Verification items for this drawing (mm, ordinates from the low corner). A direction names the side the tool comes from. Round coordinates to 2 decimals unless told otherwise and drop trailing zeros. Loops run counter-clockwise (first coordinate to the right, second up) from the corner with the lowest first, then second, coordinate; pieces in that order, holes last. Notation, with made-up numbers: M 83.5,6.5 L 87.5,6.5 A20 ccw 87.5,11.5 Z; hole C 32,13 d4. An arc over 180 degrees is marked long. One line per item, written item: value.
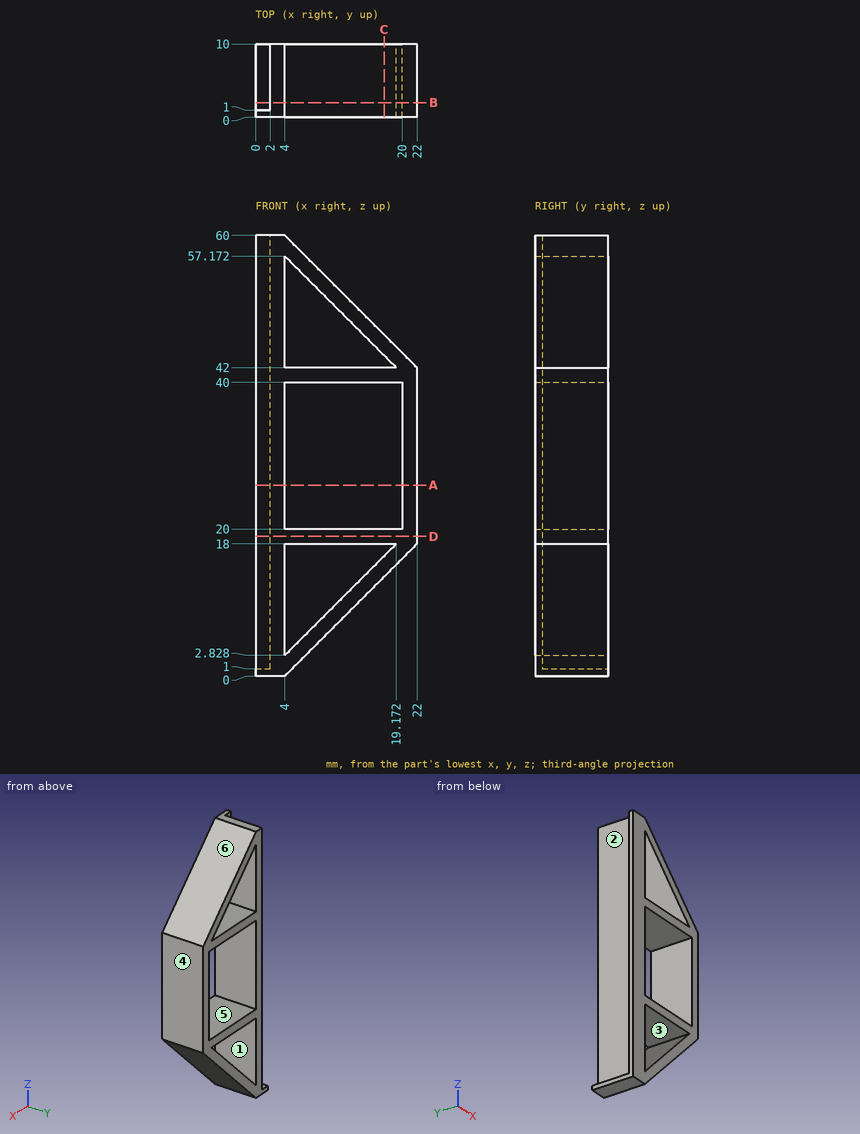
(1) Sectioned sample at B-B on y = 2. Enter the section's corners in (x, z), and give its area (3 significant figures).
Completed:
outline: M 0,0 L 4,0 L 22,18 L 22,42 L 4,60 L 2,60 L 2,1 L 0,1 Z; hole M 4,2.83 L 19.17,18 L 4,18 Z; hole M 4,20 L 20,20 L 20,40 L 4,40 Z; hole M 4,42 L 19.17,42 L 4,57.17 Z
area: 328 mm^2
(2) Thickness scan on L1, parallel to X at y = 8.75, z = 34; L2, parallel to Z at x = 14.5, y = 8.75; L3, parallel to Z at x = 10.25, y = 4.75. Record the ranges inside material, lowest first. Write a range as from..to.
Completed:
L1: x = 2..4, 20..22
L2: z = 10.5..13.33, 18..20, 40..42, 46.67..49.5
L3: z = 6.25..9.08, 18..20, 40..42, 50.92..53.75
(3) Sectioned sample at D-D on z = 19. Enter the section's corners in (x, y).
Completed:
outline: M 0,0 L 22,0 L 22,10 L 2,10 L 2,1 L 0,1 Z
(4) Mould release check, pull along Z, two halves, no side actions. Record for the marked faces 3, 4, 5 and 6: +Z half, -Z half, draft (parallel to the pull), parting line (faces both ways), or undercut.
Completed:
face 3: undercut
face 4: draft
face 5: undercut
face 6: +Z half
(5) Sectioned sample at A-A on z = 26. Enter the section's corners in (x, y).
Completed:
outline: M 0,0 L 4,0 L 4,10 L 2,10 L 2,1 L 0,1 Z; M 20,0 L 22,0 L 22,10 L 20,10 Z
(6) Depth check by flat-ended pin: pin 1 Ø0.6 at (x, y) = (1, 6) entering from +Z; pin 2 Ø1.5 at (x, y) = (10.5, 3) entering from +Z; pin 3 Ø6 at (x, y) = (13, 6.5) entering from +Z. Enter the tip coordinate at first touch or a pass-through.
Completed:
pin 1: stops at z = 1
pin 2: stops at z = 54.25
pin 3: stops at z = 54
(7) Tool access check on the marked faces 1 and 2. Record the directions out of +Z, -Z, +X, -X, +Y, -Y that give a thin tool (end or side, any length) a straight path to the whole face; none if there is none.
Completed:
face 1: +Y, -Y
face 2: +Z, -X, +Y
(8) Sectioned sample at C-C on x = 17.5. Enter the section's corners in (y, z).
Completed:
outline: M 0,13.5 L 10,13.5 L 10,16.33 L 0,16.33 Z; M 0,18 L 10,18 L 10,20 L 0,20 Z; M 0,40 L 10,40 L 10,42 L 0,42 Z; M 0,43.67 L 10,43.67 L 10,46.5 L 0,46.5 Z
